Read the model definition and answer for the solid it produces. Units are mm, in the model's axes. Face numbers are marked on the shaded views. A direction names the side the tool comes from. Give positions to 0.01 mm unless a question says otherwise; leave off trailing zeros. Write each loop counter-clockwise with the first axis right and the second up, starting at its lowest first coordinate (ties: lowest second). Pieces come first, ordered by that corner, then holes. Notation, with made-up numbers: (-36.5, 77) - (20.5, 77) arc R18 cw to (20.5, 87) - close; hole circle Ø4 at (79, 55.5). An arc over 180 degrees is marked (long way). Answer as CSV lines item,"result".
```python
from build123d import *

# Parameters (mm, degrees)
SKETCH1_R           = 1.5
BOSS_EXTRUDE1_DEPTH = 45.72
CUT_EXTRUDE1_DEPTH  = 25.4


with BuildPart() as part:
    # Sketch1 → Boss-Extrude1 (new body)
    with BuildSketch(Plane.XY):
        with BuildLine():
            Line((8.882163561, 22.821280576), (6.691616477, 10.968396178))
            ThreePointArc((6.691616477, 10.968396178), (5.818586392, 9.477556184), (4.19391315, 8.89))
            Line((4.19391315, 8.89), (2.54, 8.89))
            ThreePointArc((2.54, 8.89), (0.743948776, 8.146051224), (0, 6.35))
            Line((0, 6.35), (0, 2.54))
            ThreePointArc((0, 2.54), (0.743948776, 0.743948776), (2.54, 0))
            Line((2.54, 0), (10.16, 0))
            ThreePointArc((10.16, 0), (11.956051224, 0.743948776), (12.7, 2.54))
            Line((12.7, 2.54), (12.7, 27.94))
            ThreePointArc((12.7, 27.94), (11.956051224, 29.736051224), (10.16, 30.48))
            Line((10.16, 30.48), (2.54, 30.48))
            ThreePointArc((2.54, 30.48), (0.743948776, 29.736051224), (0, 27.94))
            Line((0, 27.94), (0, 24.13))
            ThreePointArc((0, 24.13), (1.636464911, 22.336730574), (3.571576672, 23.802737092))
            ThreePointArc((3.571576672, 23.802737092), (6.717598374, 25.967302278), (8.882163561, 22.821280576))
        make_face()
        with Locations((4.965459901, 4.445)):
            Circle(SKETCH1_R, mode=Mode.SUBTRACT)
    extrude(amount=BOSS_EXTRUDE1_DEPTH)

    # Sketch2 → Cut-Extrude1 (cut)
    with BuildSketch(Plane(origin=(12.7, 0, 0), x_dir=(0, 0, -1), z_dir=(1, 0, 0))):
        with BuildLine():
            Line((-40.64, 0), (-5.08, 0))
            Line((-5.08, 0), (-5.08, 16.51))
            ThreePointArc((-5.08, 16.51), (-5.823948776, 18.306051224), (-7.62, 19.05))
            Line((-7.62, 19.05), (-38.1, 19.05))
            ThreePointArc((-38.1, 19.05), (-39.896051224, 18.306051224), (-40.64, 16.51))
            Line((-40.64, 16.51), (-40.64, 0))
        make_face()
    extrude(amount=-CUT_EXTRUDE1_DEPTH, mode=Mode.SUBTRACT)


solid = part.part
```
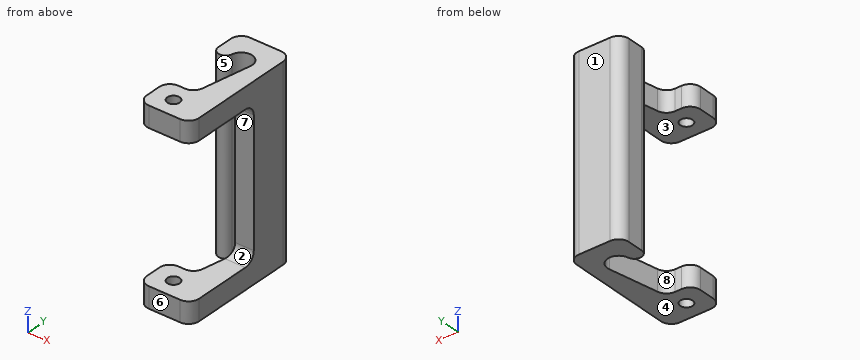
(1) A cutting plane is placed at D-D (x = 1.75). Write down the section's boundary in (y, z), and give its area (3 significant figures).
Worked out:
outline,"(0.13, 0) - (8.76, 0) - (8.76, 5.08) - (0.13, 5.08) - close; (0.13, 40.64) - (8.76, 40.64) - (8.76, 45.72) - (0.13, 45.72) - close; (22.33, 0) - (30.35, 0) - (30.35, 45.72) - (22.33, 45.72) - close"
area,"455 mm^2"
(2) The mould has two halves that part along Z. Classify the marked faces 1, 2, 3 and 4: +Z half, -Z half, draft (parallel to the pull), parting line (faces both ways), or undercut.
Worked out:
face 1,"draft"
face 2,"undercut"
face 3,"undercut"
face 4,"-Z half"
(3) A cutting plane is placed at A-A (y = 10). Write down the section's boundary in (x, z), and give its area (3 significant figures).
Worked out:
outline,"(6.29, 0) - (12.7, 0) - (12.7, 5.08) - (6.29, 5.08) - close; (6.29, 40.64) - (12.7, 40.64) - (12.7, 45.72) - (6.29, 45.72) - close"
area,"65.1 mm^2"
(4) Each of these flat-tipped pins is pushed along its axis until it touches: P1, Ø2.5, axis at x = 11, z = 27, coming from the -Y side; P2, Ø2.5, axis at x = 4.97, y = 4.44, coming from the -Z side. Where does it stop, or does it pass through?
Worked out:
P1,"stops at y = 19.05"
P2,"passes through"
(5) Find the intervals of material crossed by L1, parallel to Z at x = 10.75, y = 12; L2, parallel to X at y = 5, z = 3.5; L3, parallel to Y at x = 6, z = 4.5, in increasing order.
Worked out:
L1,"z = 0 to 5.08, 40.64 to 45.72"
L2,"x = 0 to 3.57, 6.36 to 12.7"
L3,"y = 0 to 3.36, 5.53 to 9.64, 26 to 30.48"
(6) For the marked faces 5, 6, 7 and 8, determine the directions among +Z, -Z, +X, -X, +Y, -Y from which every point of the face is accessible in a straight line to the end or side of a thin tool.
Worked out:
face 5,"+Z, -Z"
face 6,"+Z, -Z, +X, -X, -Y"
face 7,"+X, -X, -Y"
face 8,"+Z, -Z, -X"
(7) A cutting plane is placed at C-C (z = 3). Write down the section's boundary in (x, y) (3 decimals), and give its area (3 significant figures).
Worked out:
outline,"(0, 2.54) arc R2.54 ccw to (2.54, 0) - (10.16, 0) arc R2.54 ccw to (12.7, 2.54) - (12.7, 27.94) arc R2.54 ccw to (10.16, 30.48) - (2.54, 30.48) arc R2.54 ccw to (0, 27.94) - (0, 24.13) arc R1.801 ccw to (3.572, 23.803) arc R2.7 cw to (8.882, 22.821) - (6.692, 10.968) arc R2.54 cw to (4.194, 8.89) - (2.54, 8.89) arc R2.54 ccw to (0, 6.35) - close; hole circle Ø3 at (4.965, 4.445)"
area,"255 mm^2"
(8) A cutting plane is placed at B-B (x = 5.5). Write down the section's boundary in (y, z), and give its area (3 significant figures).
Worked out:
outline,"(0, 0) - (3.04, 0) - (3.04, 5.08) - (0, 5.08) - close; (0, 40.64) - (3.04, 40.64) - (3.04, 45.72) - (0, 45.72) - close; (5.85, 0) - (9.25, 0) - (9.25, 5.08) - (5.85, 5.08) - close; (5.85, 40.64) - (9.25, 40.64) - (9.25, 45.72) - (5.85, 45.72) - close; (25.91, 0) - (30.48, 0) - (30.48, 45.72) - (25.91, 45.72) - close"
area,"274 mm^2"
